from build123d import *

# Parameters (mm, degrees)
SKETCH076_R           = 12.5
PAD031_DEPTH          = 10
SKETCH077_R           = 25
PAD032_DEPTH          = 4
POCKET030_DEPTH       = 5
POLARPATTERN005_COUNT = 4


with BuildPart() as part:
    # Sketch076 → Pad031 (new body)
    with BuildSketch(Plane.XY):
        Circle(SKETCH076_R)
    extrude(amount=PAD031_DEPTH)

    # Sketch077 (on Face2 of Pad031) → Pad032 (join)
    with BuildSketch(Plane(origin=(0, 0, 0), x_dir=(1, 0, 0), z_dir=(0, 0, -1))):
        Circle(SKETCH077_R)
    extrude(amount=PAD032_DEPTH)

    # Sketch078 (on Face2 of Pad032) → Pocket030 (cut)
    with BuildSketch(Plane.XY):
        with BuildLine():
            ThreePointArc((-14.949749, 17.071067), (-17.071069, 17.071067), (-17.071069, 14.949746))
            Line((-17.071069, 14.949746), (-11.06066, 8.93934))
            ThreePointArc((-11.06066, 8.93934), (-8.93934, 8.93934), (-8.93934, 11.06066))
            Line((-14.949749, 17.071067), (-8.93934, 11.06066))
        make_face()
    pocket030 = extrude(amount=-POCKET030_DEPTH, mode=Mode.SUBTRACT)

    # PolarPattern005: Pocket030 ×4 about axis
    polarpattern005_axis = Axis((0, 0, 0), (0, 0, 1))
    for i in range(1, POLARPATTERN005_COUNT):
        add(pocket030.rotate(polarpattern005_axis, i * 360 / POLARPATTERN005_COUNT), mode=Mode.SUBTRACT)


with BuildPart() as part_1:
    # Body006 placement: moved
    add(part.part.moved(Location((260, 0, 53))))


solid = part_1.part
The model under review builds one solid part; all positions refer to its coordinate system, in mm. A direction names the side the tool comes from. Round coordinates to 2 decimals unless told otherwise and drop trailing zeros. Loops run counter-clockwise (first coordinate to the right, second up) from the corner with the lowest first, then second, coordinate; pieces in that order, holes last. Notation, with made-up numbers: (75.25, 35) -> (116.25, 35) arc R31 cw to (116.25, 64) -> close; hole circle Ø9 at (-2.5, 51). An arc over 180 degrees is marked (long way). Return JSON: item names as keys, results as strings.
(1) For faces 1 (the flat face through (245.89, -11.99, 51.03)), 2 (the flat face through (260, 0, 49)), list the 3-axis set-ups (+Z, -Z, +X, -X, +Y, -Y) from which the entire face can be reached by the end or side of a thin tool; tool diameter is ignored.
Solved:
{"face 1": "+Z, -Z", "face 2": "-Z, +X, -X, +Y, -Y"}
(2) Add section B-B on y = -10. Write out the cut boundary in (x, z), plus the area to 3 significant figures.
Solved:
{"outline": "(237.09, 49) -> (247.88, 49) -> (247.88, 53) -> (237.09, 53) -> close; (251.5, 49) -> (268.5, 49) -> (268.5, 53) -> (267.5, 53) -> (267.5, 63) -> (252.5, 63) -> (252.5, 53) -> (251.5, 53) -> close; (272.12, 49) -> (282.91, 49) -> (282.91, 53) -> (272.12, 53) -> close", "area": "304 mm2"}
(3) Add section D-D on y = 1. Write out the cut boundary in (x, z), plus the area to 3 significant figures.
Solved:
{"outline": "(235.02, 49) -> (284.98, 49) -> (284.98, 53) -> (272.46, 53) -> (272.46, 63) -> (247.54, 63) -> (247.54, 53) -> (235.02, 53) -> close", "area": "449 mm2"}
(4) Add section C-C on x = 270. Write out the cut boundary in (y, z).
Solved:
{"outline": "(-22.91, 49) -> (-12.12, 49) -> (-12.12, 53) -> (-22.91, 53) -> close; (-8.5, 49) -> (8.5, 49) -> (8.5, 53) -> (7.5, 53) -> (7.5, 63) -> (-7.5, 63) -> (-7.5, 53) -> (-8.5, 53) -> close; (12.12, 49) -> (22.91, 49) -> (22.91, 53) -> (12.12, 53) -> close"}
(5) The part is to be moulded in two halves that separate along X. For faces 3 (the cylindrical face through (271.923, 3.755, 57.93)), 4 (the cylindrical face through (251.08, -8.96, 51.03)), 5 (the flat face through (248.5, -5.9, 53)), say which applies: released by +X, released by -X, zero draft, split by the parting line, or undercut.
Solved:
{"face 3": "split by the parting line", "face 4": "undercut", "face 5": "zero draft"}
(6) For line 1 (X direction, y = 17, z = 50.75); line 2 (Y direction, x = 276.5, z = 49.5); line 3 (X direction, y = 15, z = 51.75), list the stretches that pass through material, from the lowest coordinate up.
Solved:
{"line 1": "241.67 to 242.86, 245.12 to 274.88, 277.14 to 278.33", "line 2": "-18.78 to -17.43, -14.38 to 14.38, 17.43 to 18.78", "line 3": "240 to 242.88, 247.12 to 272.88, 277.12 to 280"}
(7) For pin 1 (6 mm diameter, centred on y = 4.5, z = 58, fed in from +X); pin 2 (4 mm diameter, centred on x = 262, z = 53, fed in from +Y); pin 3 (1.5 mm diameter, centred on y = -7.5, z = 57.5, fed in from -X), all flat-tipped, find the tip position at first contact; note any pin that passes through.
Solved:
{"pin 1": "x = 272.41", "pin 2": "y = 25", "pin 3": "x = 249.48"}
(8) Add section A-A on x = 260. Write out the cut boundary in (y, z).
Solved:
{"outline": "(-25, 49) -> (25, 49) -> (25, 53) -> (12.5, 53) -> (12.5, 63) -> (-12.5, 63) -> (-12.5, 53) -> (-25, 53) -> close"}
